Design review of the part built by this model. Coordinates are the model's own, in mm. Face numbers are marked on the shaded views. A direction names the side the tool comes from. Coordinates: 2 decimals unless noted, no trailing zeros. Write each loop counter-clockwise with the first axis right and the second up, starting at its lowest first coordinate (ties: lowest second). Pieces come first, ordered by that corner, then holes.
Q1. To check wall thickness, follow probe 1 along X at (y, z) = (17.5, -3.75); probe 2 along Y at (x, z) = (35.5, -5.25); probe 3 along Y at (x, z) = (7.5, -2). State the ranges of each line that lie inside material, in increasing order.
Q2. Add section B-B, the plane x = 1. Give the boundary of the cut face in (y, z).
Q3. Machinability: for the marked faces 4, 5, 6 and 7, which of the approach directions +Z, -Z, +X, -X, +Y, -Y give a long, thin tool a straight path to every point of the face, cutting with its end or side? Answer none if there is none.
Q4. Add section C-C, the plane y = 10.5. Give the boundary of the cut face in (x, z), plus the area to 3 significant figures.
Q5. The part is to be moulded in two halves that separate along X. For the marked faces 1, 2 and 3, say which applies: +X half, -X half, draft (parallel to the pull), parting line (faces both ways), or undercut.
Q6. Add section A-A, the plane z = -1.25. Give the boundary of the cut face in (x, y).
Q7. Clearance check with flat-ended pins moving along their axes: pin 1 Ø1 at (x, y) = (23.5, 10.5) entering from +Z; pin 2 Ø8 at (x, z) = (41, -5.5) entering from -Y; pin 3 Ø1.5 at (x, z) = (31.5, -14.5) entering from +Y; pin 4 Ø6 at (y, z) = (17, -10) entering from +X. State where each tip first meets the part, or that it passes through.
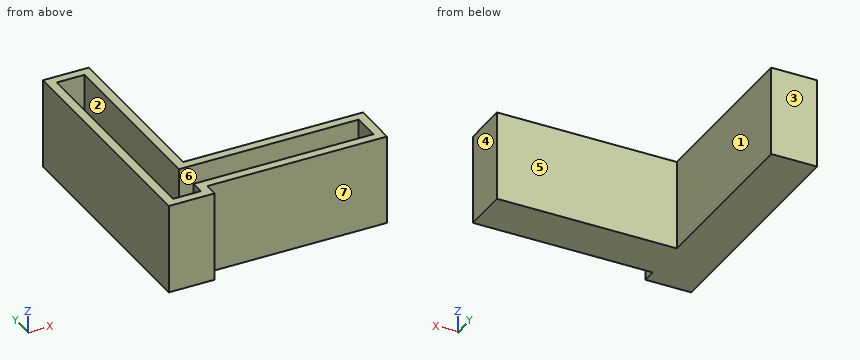
from build123d import *

# Parameters (mm, degrees)
F1_W     = 50.2
F1_H     = 53.3
F2_DEPTH = 20
F3_DEPTH = 14
F4_W     = 40
F4_H     = 40
F4_H_2   = 3.1
F5_DEPTH = 20.001


# Not quite as in the source:
# - a feature of the source that left no trace in its solid (it failed there, or was rolled back) is left out


with BuildPart() as f2:
    # F1 (on Top) → F2 (new body)
    with BuildSketch(Plane.XY):
        with Locations((23.1, 24.65)):
            Rectangle(F1_W, F1_H)
    extrude(amount=-F2_DEPTH)

    # F0 (on Top) → F3 (cut)
    with BuildSketch(Plane.XY):
        Polygon((6.2, 49.3), (0, 49.3), (0, 0), (6.2, 0), (6.2, 3.1), (46.2, 3.1), (46.2, 9.3), (6.2, 9.3), align=None)
    extrude(amount=-F3_DEPTH, mode=Mode.SUBTRACT)

    # F4 (on face) → F5 (cut, through all)
    with BuildSketch(Plane.XY):
        with Locations((28.2, 31.3)):
            Rectangle(F4_W, F4_H)
        with Locations((28.2, -0.45)):
            Rectangle(F4_W, F4_H_2)
    extrude(amount=-F5_DEPTH, mode=Mode.SUBTRACT)


solid = f2.part
Here are the results:
1. probe 1: x = -2 to 0, 6.2 to 8.2
1. probe 2: y = 1.1 to 3.1, 9.3 to 11.3
1. probe 3: y = -2 to 3.1, 9.3 to 51.3
2. outline: (-2, -20) - (51.3, -20) - (51.3, 0) - (49.3, 0) - (49.3, -14) - (0, -14) - (0, 0) - (-2, 0) - close
3. face 4: +Z, -Z, +X, +Y, -Y
3. face 5: +Z, -Z, +X, +Y
3. face 6: +Z
3. face 7: +Z, -Z, +X, -Y
4. outline: (-2, -20) - (48.2, -20) - (48.2, 0) - (6.2, 0) - (6.2, -14) - (0, -14) - (0, 0) - (-2, 0) - close
4. area: 917 mm2
5. face 1: +X half
5. face 2: undercut
5. face 3: draft
6. outline: (-2, -2) - (8.2, -2) - (8.2, 1.1) - (48.2, 1.1) - (48.2, 11.3) - (8.2, 11.3) - (8.2, 51.3) - (-2, 51.3) - close; hole (0, 0) - (6.2, 0) - (6.2, 3.1) - (46.2, 3.1) - (46.2, 9.3) - (6.2, 9.3) - (6.2, 49.3) - (0, 49.3) - close
7. pin 1: stops at z = 0
7. pin 2: stops at y = 1.1
7. pin 3: stops at y = 11.3
7. pin 4: stops at x = 8.2
